Read the model definition and answer for the solid it produces. Units are mm, in the model's axes. A direction names the side the tool comes from. Coordinates: 2 decimals unless noted, no trailing zeros. Write each loop counter-clockwise with the first axis right and the second up, starting at its lowest first coordinate (ties: lowest second). Pieces come first, ordered by that corner, then holes. Notation, with made-up numbers: (35, 39) -> (71, 39) arc R8 ccw to (71, 50) -> close; hole circle Ø4 at (-35, 43). An arc over 180 degrees is marked (long way). One line per item, written item: value. Start each with the question number.
from build123d import *

# Parameters (mm, degrees)
F0_R           = 4.1275
F0_R_2         = 6.35
F1_DEPTH       = 15.875
F3_D           = 8.255
F3_CSINK_D     = 15.24
F3_CSINK_ANGLE = 90


with BuildPart() as f1:
    # F0 (on Front) → F1 (new body)
    with BuildSketch(Plane.XZ):
        with BuildLine():
            Line((-27.029276, -56.007), (0, -56.007))
            Line((0, -56.007), (27.029276, -56.007))
            ThreePointArc((27.029276, -56.007), (28.197928, -55.982797), (29.36658, -56.007))
            ThreePointArc((29.36658, -56.007), (47.874791, -63.97181), (56.35625, -82.249034))
            Line((56.35625, -82.249034), (56.35625, -89.3445))
            Line((56.35625, -89.3445), (72.23125, -89.3445))
            Line((72.23125, -89.3445), (72.23125, -70.2945))
            Line((72.23125, -70.2945), (72.073391, -51.823376))
            ThreePointArc((72.073391, -51.823376), (71.871442, -48.75548), (72.020927, -45.68458))
            ThreePointArc((72.020927, -45.68458), (76.627023, -33.253211), (86.611983, -24.532223))
            ThreePointArc((86.611983, -24.532223), (91.49573, -22.630497), (96.655561, -21.711968))
            Line((96.655561, -21.711968), (127, -13.191196))
            Line((127, -13.191196), (127, -6.35))
            ThreePointArc((127, -6.35), (120.65, 0), (127, 6.35))
            Line((127, 6.35), (127, 13.484294))
            Line((127, 13.484294), (18.594601, 52.185375))
            ThreePointArc((18.594601, 52.185375), (-8.60389, 55.18782), (-33.587092, 44.024833))
            Line((-33.587092, 44.024833), (-76.257501, 10.965124))
            ThreePointArc((-76.257501, 10.965124), (-81.301476, 5.491238), (-82.411728, -1.868957))
            Line((-82.411728, -1.868957), (-72.23125, -70.2945))
            Line((-72.23125, -70.2945), (-72.23125, -89.3445))
            Line((-72.23125, -89.3445), (-56.35625, -89.3445))
            Line((-56.35625, -89.3445), (-56.35625, -86.1695))
            ThreePointArc((-56.35625, -86.1695), (-56.424398, -84.209267), (-56.35625, -82.249034))
            ThreePointArc((-56.35625, -82.249034), (-47.874791, -63.97181), (-29.36658, -56.007))
            ThreePointArc((-29.36658, -56.007), (-28.197928, -55.982797), (-27.029276, -56.007))
        make_face()
        with Locations((-37.109015, -21.4249)):
            Circle(F0_R, mode=Mode.SUBTRACT)
        with Locations((37.109015, -21.4249)):
            Circle(F0_R, mode=Mode.SUBTRACT)
        with BuildLine():
            ThreePointArc((71.462556, -28.786209), (71.668645, -28.726833), (71.875518, -28.670248))
            Line((71.875518, -28.670248), (71.462556, -28.786209))
        make_face(mode=Mode.SUBTRACT)
        with Locations((-69.85, 0)):
            Circle(F0_R_2, mode=Mode.SUBTRACT)
        with BuildLine():
            ThreePointArc((0, -34.925), (-19.48747, -28.982653), (-32.343511, -13.177743))
            ThreePointArc((-32.343511, -13.177743), (-6.714108, 34.273552), (34.925, 0))
            ThreePointArc((34.925, 0), (34.273552, -6.714108), (32.343511, -13.177743))
            ThreePointArc((32.343511, -13.177743), (19.48747, -28.982653), (0, -34.925))
        make_face(mode=Mode.SUBTRACT)
        with Locations((0, 42.8498)):
            Circle(F0_R, mode=Mode.SUBTRACT)
        with BuildLine():
            Line((-29.36658, -56.007), (-27.029276, -56.007))
            ThreePointArc((-27.029276, -56.007), (-28.197928, -55.982797), (-29.36658, -56.007))
        make_face()
        with BuildLine():
            ThreePointArc((29.36658, -56.007), (28.197928, -55.982797), (27.029276, -56.007))
            Line((27.029276, -56.007), (29.36658, -56.007))
        make_face()
        with BuildLine():
            Line((-56.35625, -86.1695), (-56.35625, -82.249034))
            ThreePointArc((-56.35625, -82.249034), (-56.424398, -84.209267), (-56.35625, -86.1695))
        make_face()
        with BuildLine():
            ThreePointArc((72.020927, -45.68458), (71.871442, -48.75548), (72.073391, -51.823376))
            Line((72.073391, -51.823376), (72.020927, -45.68458))
        make_face()
        with BuildLine():
            ThreePointArc((96.655561, -21.711968), (91.49573, -22.630497), (86.611983, -24.532223))
            Line((86.611983, -24.532223), (96.655561, -21.711968))
        make_face()
        with BuildLine():
            Line((127, -6.35), (127, -13.191196))
            Line((127, -13.191196), (130.43339, -12.227094))
            ThreePointArc((130.43339, -12.227094), (139.694559, -0.371702), (131.142923, 12.005257))
            Line((131.142923, 12.005257), (127, 13.484294))
            Line((127, 13.484294), (127, 6.35))
            ThreePointArc((127, 6.35), (131.490128, 4.490128), (133.35, 0))
            ThreePointArc((133.35, 0), (131.490128, -4.490128), (127, -6.35))
        make_face()
    extrude(amount=F1_DEPTH)

    # F3 (through all)
    with Locations(Plane.XZ.offset(15.875)):
        with Locations((-37.109015, -21.4249), (0, 42.8498), (37.109015, -21.4249)):
            CounterSinkHole(F3_D / 2, F3_CSINK_D / 2, counter_sink_angle=F3_CSINK_ANGLE)


solid = f1.part
1. Given pin 1 (3 mm diameter, centred on x = 71, y = -14, fed in from +Z); pin 2 (5.5 mm diameter, centred on y = -11, z = -85, fed in from +X); pin 3 (5.5 mm diameter, centred on y = -6.5, z = -86, fed in from -X); pin 4 (10 mm diameter, centred on x = -69.85, z = 0, fed in from +Y), each flat-ended and moving along its own axis, determine where each tip first touches the part or whether it passes through.
2. For a pull along Z with two mould halves and no side action, classify faces 1 (the face through (-63.984, -7.826, -2.432)), 2 (the face through (-77.393, -7.826, -35.603)), 3 (the face through (-56.356, -8, -86)) as +Z half, -Z half, draft (parallel to the pull), parting line (faces both ways), or undercut.
3. A tool of negligible diameter and unlimited length cuts with its end or side. For faces 4 (the face through (-8.221, -7.826, 55.246)), 5 (the face through (72.231, -8, -80)), 6 (the face through (-72.231, -8, -80)), 7 (the face through (0, -8, -56.007)), from which of +Z, -Z, +X, -X, +Y, -Y can it reach the whole face along a straight path? Write none if from no direction.
4. A cutting plane is placed at B-B on z = 4. Give the vertices of the cut face in (x, y) (3 decimals), then the cut area to 3 significant figures.
5. Find the intervals of material crossed by probe 1 along X at (y, z) = (-12.5, 4); probe 2 along X at (y, z) = (-4, -83); probe 3 along Z at (x, y) = (-1.5, -8.25), in increasing order. Write a range as from..to.
6. A cutting plane is placed at A-A on x = -19. Give the vertices of the cut face in (y, z) (3 decimals).
Derived:
1. pin 1: stops at z = 34.01
1. pin 2: stops at x = 72.23
1. pin 3: stops at x = -72.23
1. pin 4: passes through
2. face 1: undercut
2. face 2: -Z half
2. face 3: draft
3. face 4: +Z, +Y, -Y
3. face 5: -Z, +X, +Y, -Y
3. face 6: -Z, -X, +Y, -Y
3. face 7: -Z, +Y, -Y
4. outline: (-81.904, -15.875) -> (-74.782, -15.875) -> (-74.782, 0) -> (-81.904, 0) -> close; (-64.918, -15.875) -> (-34.695, -15.875) -> (-34.695, 0) -> (-64.918, 0) -> close; (34.695, -15.875) -> (122.068, -15.875) -> (122.068, 0) -> (34.695, 0) -> close; (131.932, -15.875) -> (139.054, -15.875) -> (139.054, 0) -> (131.932, 0) -> close
4. area: 2,090 mm2
5. probe 1: x = -81.9..-74.78, -64.92..-34.7, 34.7..122.07, 131.93..139.05
5. probe 2: x = -72.23..-56.36, 56.36..72.23
5. probe 3: z = -56.01..-34.89, 34.89..39, 46.7..55.81
6. outline: (-15.875, -56.007) -> (0, -56.007) -> (0, -29.305) -> (-15.875, -29.305) -> close; (-15.875, 29.305) -> (0, 29.305) -> (0, 52.442) -> (-15.875, 52.442) -> close
